Source: three-view drawing plus pictorial views. Frame: mm from the lowest corner of the part. Round coordinates to 2 decimals unless told otherwise and drop trailing zeros. Write each loop counter-clockwise with the first axis right and the second up, starting at its lowest first coordinate (ties: lowest second). Pieces come first, ordered by that corner, then holes. Notation, with made-up numbers: (83, -25.75) - (101, -25.75) arc R22 ccw to (101, -3.75) - close; hole circle Ø6 at (44, -21). An arc over 180 degrees is marked (long way). Write each question's results on one line, items separated by ' | '.
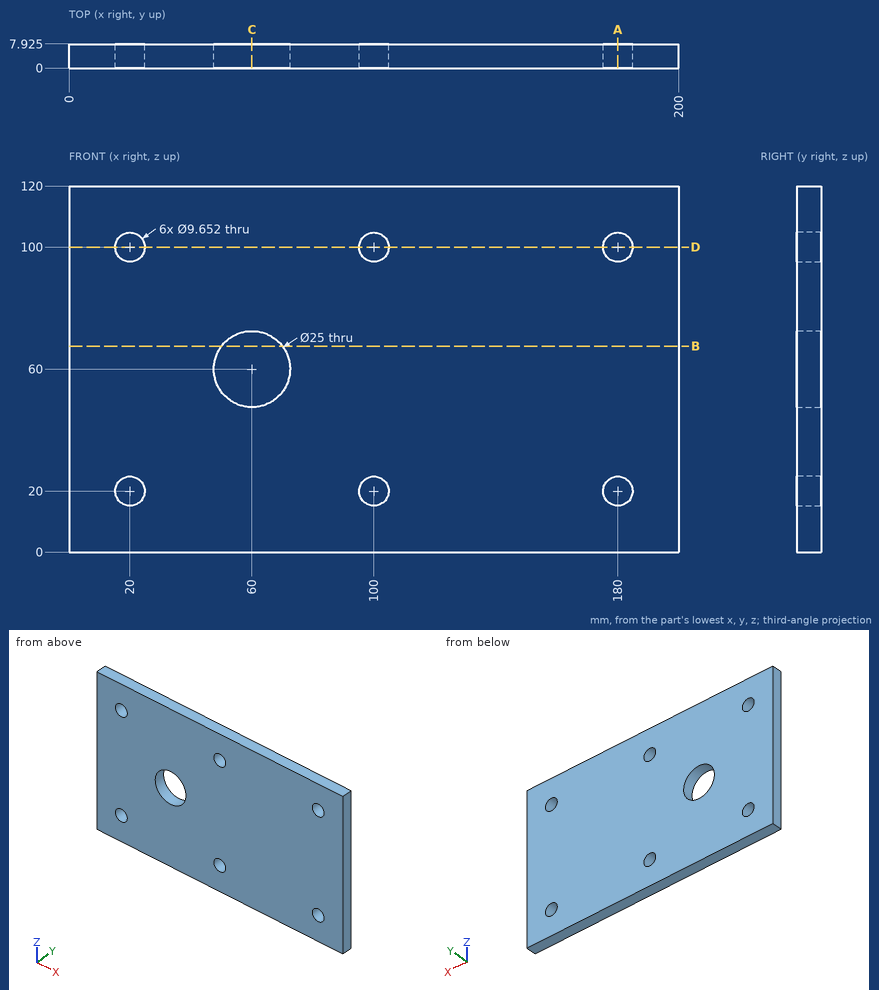
Q1. Section query D-D, the plane z = 100. Return loops of the section in (x, y) (1 decimal).
Answer block:
outline: (0, 0) - (15.2, 0) - (15.2, 7.9) - (0, 7.9) - close; (24.8, 0) - (95.2, 0) - (95.2, 7.9) - (24.8, 7.9) - close; (104.8, 0) - (175.2, 0) - (175.2, 7.9) - (104.8, 7.9) - close; (184.8, 0) - (200, 0) - (200, 7.9) - (184.8, 7.9) - close
Q2. Pin query (flat end, axial travel): pin 1 (7.5 mm diameter, centred on x = 180, z = 20, fed in from -Y); pin 2 (11 mm diameter, centred on x = 20, z = 100, fed in from -Y). Return the tip coordinate at first contact, or that it passes through.
Answer block:
pin 1: through | pin 2: y = 0
Q3. Section query C-C, the plane x = 60. Return loops of the section in (y, z) (1 decimal), plus the area to 3 significant figures.
Answer block:
outline: (0, 0) - (7.9, 0) - (7.9, 47.5) - (0, 47.5) - close; (0, 72.5) - (7.9, 72.5) - (7.9, 120) - (0, 120) - close | area: 753 mm2
Q4. Section query B-B, the plane z = 67.5. Return loops of the section in (x, y) (1 decimal).
Answer block:
outline: (0, 0) - (50, 0) - (50, 7.9) - (0, 7.9) - close; (70, 0) - (200, 0) - (200, 7.9) - (70, 7.9) - close
Q5. Ray query, line 1 along X through (y, z) = (5.25, 100); line 2 along Z through (x, y) = (180, 6.25); line 3 along X through (y, z) = (7.5, 102). Return the intervals inside material, ascending.
Answer block:
line 1: 0 to 15.17, 24.83 to 95.17, 104.83 to 175.17, 184.83 to 200 | line 2: 0 to 15.17, 24.83 to 95.17, 104.83 to 120 | line 3: 0 to 15.61, 24.39 to 95.61, 104.39 to 175.61, 184.39 to 200
Q6. Section query A-A, the plane x = 180. Return loops of the section in (y, z) (1 decimal).
Answer block:
outline: (0, 0) - (7.9, 0) - (7.9, 15.2) - (0, 15.2) - close; (0, 24.8) - (7.9, 24.8) - (7.9, 95.2) - (0, 95.2) - close; (0, 104.8) - (7.9, 104.8) - (7.9, 120) - (0, 120) - close
